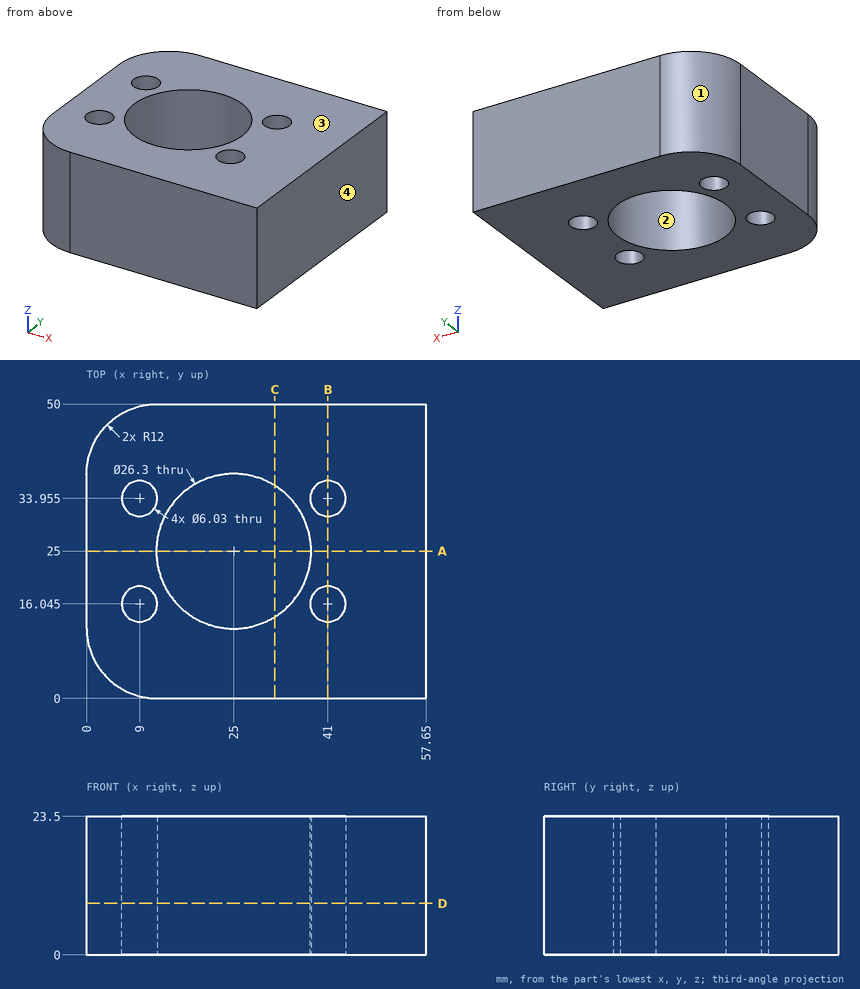
Geometry: see drawing. Coordinates: mm, zero at the bounding-box minimum. Give positions to 0.01 mm unless a question says otherwise; leave off trailing zeros. Order: outer loops, then holes, each group sorted by start corner. A loop starts at its lowest first (then second) coordinate and runs counter-clockwise, first axis right, second up. Notation, with made-up numbers: (63.25, -18.5) - (73.25, -18.5) arc R21 ccw to (73.25, 7.5) - close; hole circle Ø1 at (19.25, 61). An arc over 180 degrees is marked (long way). Use a Markdown table: item, result.
(1) Section query C-C (x = 32). Output: boundary loops of the cut face in (y, z).
Computed values:
| item | result |
|---|---|
| outline | (0, 0) - (13.87, 0) - (13.87, 23.5) - (0, 23.5) - close; (36.13, 0) - (50, 0) - (50, 23.5) - (36.13, 23.5) - close |
(2) Pin query (flat end, axial travel): pin 1 (3.5 mm diameter, centred on x = 9, y = 33.955, fed in from +Z). Return the tip coordinate at first contact, or that it passes through.
Computed values:
| item | result |
|---|---|
| pin 1 | passes through |
(3) Section query D-D (z = 8.75). Output: boundary loops of the cut face in (x, y) (3 decimals).
Computed values:
| item | result |
|---|---|
| outline | (0, 12) arc R12 ccw to (12, 0) - (57.65, 0) - (57.65, 50) - (12, 50) arc R12 ccw to (0, 38) - close; hole circle Ø6.03 at (9, 16.045); hole circle Ø6.03 at (9, 33.955); hole circle Ø26.3 at (25, 25); hole circle Ø6.03 at (41, 16.045); hole circle Ø6.03 at (41, 33.955) |
(4) Section query A-A (y = 25). Output: boundary loops of the cut face in (x, z), then the cut area to 3 significant figures.
Computed values:
| item | result |
|---|---|
| outline | (0, 0) - (11.85, 0) - (11.85, 23.5) - (0, 23.5) - close; (38.15, 0) - (57.65, 0) - (57.65, 23.5) - (38.15, 23.5) - close |
| area | 737 mm2 |
(5) Line query: line 1 (Y direction, x = 41, z = 17.75); line 2 (Y direction, x = 9, z = 10.5); line 3 (X direction, y = 14.5, z = 9.25). Output: solid intervals per line, ascending. Write a range as from..to.
Computed values:
| item | result |
|---|---|
| line 1 | y = 0..13.03, 19.06..30.94, 36.97..50 |
| line 2 | y = 0.38..13.03, 19.06..30.94, 36.97..49.62 |
| line 3 | x = 0..6.41, 11.59..17.08, 32.92..38.41, 43.59..57.65 |
(6) Section query B-B (x = 41). Output: boundary loops of the cut face in (y, z).
Computed values:
| item | result |
|---|---|
| outline | (0, 0) - (13.03, 0) - (13.03, 23.5) - (0, 23.5) - close; (19.06, 0) - (30.94, 0) - (30.94, 23.5) - (19.06, 23.5) - close; (36.97, 0) - (50, 0) - (50, 23.5) - (36.97, 23.5) - close |
(7) Draft query along X for the marked faces 1, 2, 3 and 4. Return one class per face: released by +X, released by -X, zero draft, split by the parting line, or undercut.
Computed values:
| item | result |
|---|---|
| face 1 | released by -X |
| face 2 | undercut |
| face 3 | zero draft |
| face 4 | released by +X |
